The listing builds one solid part. Answer for the finished solid, in the listing's coordinates (mm). Face numbers are marked on the shaded views. A direction names the side the tool comes from. Coordinates: 2 decimals unless noted, no trailing zeros. Order: outer loops, then holes, each group sorted by start corner. A loop starts at its lowest first (then second) coordinate and runs counter-clockwise, first axis right, second up. Notation, with made-up numbers: (26, 68.5) -> (76, 68.5) arc R26 cw to (76, 106.5) -> close; hole circle Ø11 at (-26, 34). An arc over 180 degrees is marked (long way). Return JSON: item names as keys, results as strings.
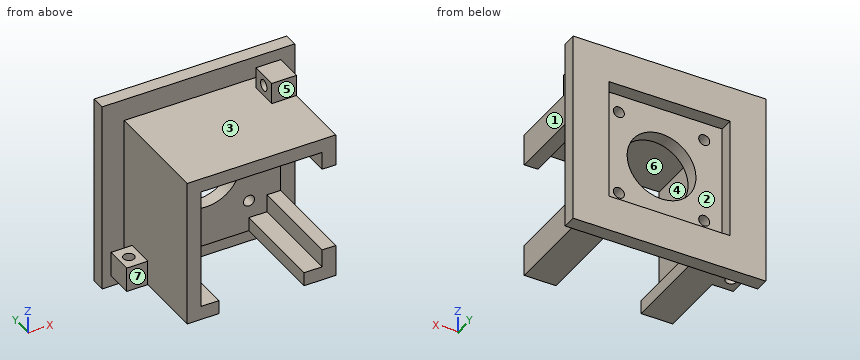
```python
from build123d import *

# Parameters (mm, degrees)
EXTRUDE_1_DEPTH          = 10
EXTRUDE_1_DEPTH_BACK     = 35
SKETCH_1_W               = 56
SKETCH_1_H               = 56
SKETCH_1_W_2             = 44
SKETCH_1_H_2             = 44
SKETCH_3_W               = 70
SKETCH_3_H               = 70
SKETCH_3_W_2             = 54
SKETCH_3_H_2             = 54
EXTRUDE_2_DEPTH          = 10
CUT_EXTRUDE_1_DEPTH      = 5
CUT_EXTRUDE_1_DEPTH_BACK = 40
SKETCH_3_2_W             = 70
SKETCH_3_2_H             = 70
SKETCH_3_2_W_2           = 54
SKETCH_3_2_H_2           = 54
SKETCH_4_W               = 47.606985224
SKETCH_4_H               = 48.466705047
SKETCH_4_R               = 12.5
SKETCH_4_R_2             = 2
EXTRUDE_3_DEPTH          = 5
CUT_EXTRUDE_2_DEPTH      = 50
SKETCH_6_W               = 12.5
SKETCH_6_H               = 9
SKETCH_6_W_2             = 9
SKETCH_6_H_2             = 12.5
EXTRUDE_4_DEPTH          = 10
SKETCH_7_R               = 2
CUT_EXTRUDE_3_DEPTH      = 1000
SKETCH_8_R               = 2
CUT_EXTRUDE_4_DEPTH      = 1000


with BuildPart() as part:
    # Sketch 1 → Extrude 1 (new, two sides: drawn at the far end of the back side and taken through both)
    with BuildSketch(Plane(origin=(0, 0, 0), x_dir=(1, 0, 0), z_dir=(0, 1, 0)).offset(-EXTRUDE_1_DEPTH_BACK)):
        Rectangle(SKETCH_1_W, SKETCH_1_H)
        Rectangle(SKETCH_1_W_2, SKETCH_1_H_2, mode=Mode.SUBTRACT)
    extrude(amount=EXTRUDE_1_DEPTH + EXTRUDE_1_DEPTH_BACK)

    # Sketch 3 → Extrude 2 (add)
    with BuildSketch(Plane(origin=(0, 0, 0), x_dir=(1, 0, 0), z_dir=(0, 1, 0))):
        Rectangle(SKETCH_3_W, SKETCH_3_H)
        Rectangle(SKETCH_3_W_2, SKETCH_3_H_2, mode=Mode.SUBTRACT)
    extrude(amount=EXTRUDE_2_DEPTH)

    # Sketch 3_2 → Cut-Extrude 1 (cut, two sides: drawn at the far end of the back side and taken through both)
    with BuildSketch(Plane(origin=(0, 0, 0), x_dir=(1, 0, 0), z_dir=(0, 1, 0)).offset(-CUT_EXTRUDE_1_DEPTH_BACK)):
        Rectangle(SKETCH_3_2_W, SKETCH_3_2_H)
        Rectangle(SKETCH_3_2_W_2, SKETCH_3_2_H_2, mode=Mode.SUBTRACT)
    extrude(amount=CUT_EXTRUDE_1_DEPTH + CUT_EXTRUDE_1_DEPTH_BACK, mode=Mode.SUBTRACT)

    # Sketch 4 → Extrude 3 (add)
    with BuildSketch(Plane(origin=(0, 0, 0), x_dir=(1, 0, 0), z_dir=(0, 1, 0))):
        with Locations((0.268662445, 0.4835924)):
            Rectangle(SKETCH_4_W, SKETCH_4_H)
        with Locations(Location((0, 0, 0), (0, 0, 270))):
            Circle(SKETCH_4_R, mode=Mode.SUBTRACT)
        with Locations(Location((-15.5, 15.5, 0), (0, 0, 270))):
            Circle(SKETCH_4_R_2, mode=Mode.SUBTRACT)
        with Locations(Location((-15.5, -15.5, 0), (0, 0, 270))):
            Circle(SKETCH_4_R_2, mode=Mode.SUBTRACT)
        with Locations(Location((15.5, -15.5, 0), (0, 0, 270))):
            Circle(SKETCH_4_R_2, mode=Mode.SUBTRACT)
        with Locations(Location((15.5, 15.5, 0), (0, 0, 270))):
            Circle(SKETCH_4_R_2, mode=Mode.SUBTRACT)
    extrude(amount=EXTRUDE_3_DEPTH)

    # Sketch 5 → Cut-Extrude 2 (cut)
    with BuildSketch(Plane(origin=(0, 0, 0), x_dir=(1, 0, 0), z_dir=(0, 1, 0))):
        Polygon((-15.5, -15.5), (45.904177047, -15.5), (45.904177047, 15.5), (15.5, 15.5), (15.5, 51.810948834), (-15.5, 51.810948834), align=None)
    extrude(amount=-CUT_EXTRUDE_2_DEPTH, mode=Mode.SUBTRACT)

    # Sketch 6 → Extrude 4 (add)
    with BuildSketch(Plane(origin=(0, 0, 0), x_dir=(1, 0, 0), z_dir=(0, 1, 0))):
        with Locations((-28.3864137, 22.5)):
            Rectangle(SKETCH_6_W, SKETCH_6_H)
        with Locations((22.5, -28.484371776)):
            Rectangle(SKETCH_6_W_2, SKETCH_6_H_2)
    extrude(amount=-EXTRUDE_4_DEPTH)

    # Sketch 7 → Cut-Extrude 3 (cut)
    with BuildSketch(Plane(origin=(0, 0, 0), x_dir=(0, 0, -1), z_dir=(1, 0, 0))):
        with Locations(Location((-31, -5, 0), (0, 0, 180))):
            Circle(SKETCH_7_R)
    extrude(amount=CUT_EXTRUDE_3_DEPTH, mode=Mode.SUBTRACT)

    # Sketch 8 → Cut-Extrude 4 (cut)
    with BuildSketch(Plane.XY):
        with Locations((-31, -5)):
            Circle(SKETCH_8_R)
    extrude(amount=-CUT_EXTRUDE_4_DEPTH, mode=Mode.SUBTRACT)


solid = part.part
```
Item 1: The part is cut by section B-B on z = 31. Determine the outline of the cut face in (x, y).
Answer list:
{"outline": "(-35, 5) -> (35, 5) -> (35, 10) -> (-35, 10) -> close; (18, -10) -> (27, -10) -> (27, -7) -> (18, -7) -> close; (18, -3) -> (27, -3) -> (27, 0) -> (18, 0) -> close"}
Item 2: Flat-ended cylindrical pins translate along their axes: pin 1 (8 mm diameter, centred on y = -26, z = -7, fed in from +X); pin 2 (6 mm diameter, centred on x = -2, y = 0.5, fed in from +Z); pin 3 (20 mm diameter, centred on y = -16.5, z = 6.5, fed in from -X). Find the tip coordinate at first contact, or state that the pin passes through.
Answer list:
{"pin 1": "x = -22", "pin 2": "z = 27", "pin 3": "x = -27"}
Item 3: The part is cut by section D-D on x = 25.5. Determine the outline of the cut face in (y, z), plus the area to 3 significant figures.
Answer list:
{"outline": "(-35, -27) -> (5, -27) -> (5, -35) -> (10, -35) -> (10, 35) -> (5, 35) -> (5, 27) -> (0, 27) -> (0, 34.73) -> (-10, 34.73) -> (-10, 27) -> (-35, 27) -> (-35, 15.5) -> (0, 15.5) -> (0, -15.5) -> (-35, -15.5) -> close; hole circle Ø4 at (-5, 31)", "area": "1,490 mm2"}
Item 4: Determine the mould class of the marked faces 1, 2, 3 and 4 for opening direction X: pulls with the +X half, pulls with the -X half, needs draft (parallel to the pull), parting line crosses it, or undercut.
Answer list:
{"face 1": "pulls with the +X half", "face 2": "undercut", "face 3": "needs draft", "face 4": "undercut"}
Item 5: The part is cut by section A-A on x = 0. Determine the outline of the cut face in (y, z).
Answer list:
{"outline": "(-35, 22) -> (0, 22) -> (0, 12.5) -> (5, 12.5) -> (5, 22) -> (10, 22) -> (10, 35) -> (5, 35) -> (5, 27) -> (-35, 27) -> close; (0, -27) -> (5, -27) -> (5, -35) -> (10, -35) -> (10, -22) -> (5, -22) -> (5, -12.5) -> (0, -12.5) -> close"}
Item 6: The part is cut by section C-C on y = -5. Determine the outline of the cut face in (x, z).
Answer list:
{"outline": "(-34.64, -27) -> (-33, -27) -> (-33, -18) -> (-34.64, -18) -> close; (-29, -27) -> (-15.5, -27) -> (-15.5, -22) -> (-22, -22) -> (-22, 22) -> (22, 22) -> (22, 15.5) -> (27, 15.5) -> (27, 29) -> (18, 29) -> (18, 27) -> (-27, 27) -> (-27, -18) -> (-29, -18) -> close; (15.5, -27) -> (27, -27) -> (27, -15.5) -> (22, -15.5) -> (22, -22) -> (15.5, -22) -> close; (18, 33) -> (27, 33) -> (27, 34.73) -> (18, 34.73) -> close"}
Item 7: Which of the six approach directions +Z, -Z, +X, -X, +Y, -Y give full straight-line access (tool end or side, diameter ignored) to the marked faces 5, 6 and 7?
Answer list:
{"face 5": "+Z, +X, -X, -Y", "face 6": "-Y", "face 7": "+Z, -Z, -X, -Y"}
Item 8: Find the intervals of material crossed by probe 1 along X at (y, z) = (3.6, 15.5); probe 2 along Y at (x, z) = (20.75, 31); probe 3 along X at (y, z) = (3.35, 0), in increasing order.
Answer list:
{"probe 1": "-27 to -17.5, -13.5 to 13.5, 17.5 to 27", "probe 2": "-10 to -7, -3 to 0, 5 to 10", "probe 3": "-27 to -12.5, 12.5 to 27"}
